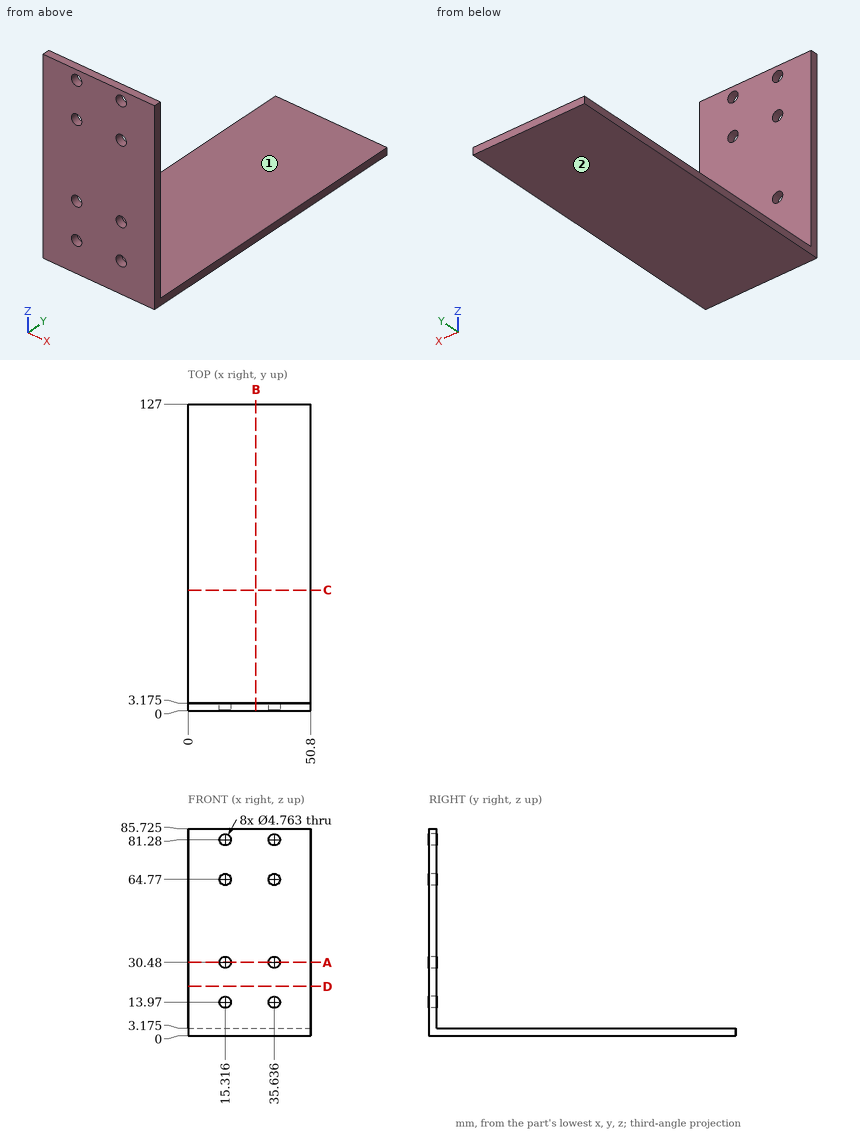
The figure shows three views and two pictorial views of one solid part (mm, origin at its lowest corner). Answer the questions. A direction names the side the tool comes from. Give positions to 0.01 mm unless a question says otherwise; leave off trailing zeros. Write each loop counter-clockwise with the first axis right and the second up, starting at its lowest first coordinate (ties: lowest second). Pieces come first, ordered by that corner, then holes. Notation, with made-up numbers: M -38,5 L -21,5 A25 cw -21,40 Z; hole C 11,-35.75 d3. An arc over 180 degrees is marked long. One line per item, written item: value. Start each with the question number.
(1) Find section C-C (y = 50). Determine the outline of the cut face in (x, z) (1 decimal), plus the area to 3 significant figures.
(2) Find the intervals of material crossed by line 1 (Y direction, x = 44, z = 19.5) (1 decimal); line 2 (X direction, y = 1, z = 64); line 3 (X direction, y = 2, z = 13), in increasing order.
(3) A tool of negligible diameter and unlimited length cuts with its end or side. For the marked faces 1 and 2, from which of +Z, -Z, +X, -X, +Y, -Y can it reach the whole face along a straight path? Write none if from no direction.
(4) Find section B-B (x = 28). Determine the outline of the cut face in (y, z) (1 decimal).
(5) A flat-ended cylindrical pin translates along its axis: pin 1 Ø15 at (x, z) = (27.5, 58) entering from +Y (3 decimals). Find the tip coordinate at first contact, or state that the pin passes through.
(6) Find section A-A (z = 30.48). Determine the outline of the cut face in (x, y) (1 decimal), plus the area to 3 significant figures.
Results below:
1. outline: M 0,0 L 50.8,0 L 50.8,3.2 L 0,3.2 Z
1. area: 161 mm^2
2. line 1: y = 0 to 3.2
2. line 2: x = 0 to 13.06, 17.57 to 33.38, 37.89 to 50.8
2. line 3: x = 0 to 13.14, 17.49 to 33.46, 37.81 to 50.8
3. face 1: +Z, +X, -X, +Y
3. face 2: -Z, +X, -X, +Y, -Y
4. outline: M 0,0 L 127,0 L 127,3.2 L 3.2,3.2 L 3.2,85.7 L 0,85.7 Z
5. pin 1: stops at y = 3.175
6. outline: M 0,0 L 12.9,0 L 12.9,3.2 L 0,3.2 Z; M 17.7,0 L 33.3,0 L 33.3,3.2 L 17.7,3.2 Z; M 38,0 L 50.8,0 L 50.8,3.2 L 38,3.2 Z
6. area: 131 mm^2
